from build123d import *

# Parameters (mm, degrees)
EXTRUDE_1_DEPTH          = 22
CUT_EXTRUDE_1_DEPTH      = 36.358874416
CUT_EXTRUDE_1_DEPTH_BACK = 36.358874416
SKETCH_3_W               = 15.710666492
SKETCH_3_H               = 11.25
SKETCH_3_W_2             = 17.010469835
SKETCH_3_H_2             = 12.25
SKETCH_4_R               = 2
CUT_EXTRUDE_2_DEPTH      = 52.983170353
PATTERN_LINEAR_1_COUNT   = 2
PATTERN_LINEAR_1_PITCH   = 23.5


with BuildPart() as part:
    # 草图1 → 凸台-拉伸1 (new, symmetric)
    with BuildSketch(Plane.XY):
        with BuildLine():
            Line((26.5, -8), (26.5, -6.486832981))
            ThreePointArc((26.5, -6.486832981), (26.461262373, -6.006286251), (26.346049894, -5.538149682))
            Line((26.346049894, -5.538149682), (25.183772234, -2.051316702))
            ThreePointArc((25.183772234, -2.051316702), (24.091853194, -0.566273444), (22.33772234, 0))
            Line((22.33772234, 0), (6.2, 0))
            ThreePointArc((6.2, 0), (-3.691899698, 4.980951377), (-1.803186005, -5.931991253))
            Line((-1.803186005, -5.931991253), (5, -8))
            Line((5, -8), (26.5, -8))
        make_face()
    extrude(amount=EXTRUDE_1_DEPTH, both=True)

    # 草图3 → 切除-拉伸1 (cut, two sides: drawn at the far end of the back side and taken through both)
    with BuildSketch(Plane(origin=(0, 0, 0), x_dir=(1, 0, 0), z_dir=(0, 1, 0)).offset(-CUT_EXTRUDE_1_DEPTH_BACK)):
        with Locations((-1.180894358, -16.375)):
            Rectangle(SKETCH_3_W, SKETCH_3_H)
        with Locations((-1.83079603, 5.625)):
            Rectangle(SKETCH_3_W_2, SKETCH_3_H_2)
    extrude(amount=CUT_EXTRUDE_1_DEPTH + CUT_EXTRUDE_1_DEPTH_BACK, mode=Mode.SUBTRACT)

    # 草图4 → 切除-拉伸2 (cut, through all)
    with BuildSketch(Plane(origin=(0, 0, -22), x_dir=(-1, 0, 0), z_dir=(0, 0, -1))):
        Circle(SKETCH_4_R)
    extrude(amount=-CUT_EXTRUDE_2_DEPTH, mode=Mode.SUBTRACT)

    # 草图5 → 切除-旋转1 (revolve, cut)
    with BuildSketch(Plane(origin=(0, 0, -11.75), x_dir=(-1, 0, 0), z_dir=(0, 0, -1))):
        Polygon((-15, 0), (-15, -8), (-11.75, -8), (-11.75, -6), (-9.2, -1), (-9.2, 0), align=None)
    cut_revolve_1 = revolve(axis=Axis((15, 0, -11.75), (0, -1, 0)), mode=Mode.SUBTRACT)

    # 阵列(线性)1: 切除-旋转1 ×2
    with Locations(*[(0, 0, i * PATTERN_LINEAR_1_PITCH) for i in range(1, PATTERN_LINEAR_1_COUNT)]):
        add(cut_revolve_1, mode=Mode.SUBTRACT)


solid = part.part
The model under review builds one solid part; all positions refer to its coordinate system, in mm. A direction names the side the tool comes from. Give positions to 0.01 mm unless a question says otherwise; leave off trailing zeros. Loops run counter-clockwise (first coordinate to the right, second up) from the corner with the lowest first, then second, coordinate; pieces in that order, holes last. Notation, with made-up numbers: (39.25, 83.5) -> (52.25, 83.5) arc R16 cw to (52.25, 87.5) -> close; hole circle Ø7 at (-8, 4). An arc over 180 degrees is marked (long way). Put each result on its own line as item: value. Start each with the question number.
1. For faces 4 (the face through (24.11, -0.58, 0.31)), 5 (the face through (0, -3, 10.75)), 6 (the face through (20.794, -0.493, 11.495)), list the 3-axis set-ups (+Z, -Z, +X, -X, +Y, -Y) from which the entire face can be reached by the end or side of a thin tool; tool diameter is ignored.
2. We need section D-D on y = 5.25. State the section outline as (x, z) points.
3. Wall thickness on probe 1 along Z at (x, y) = (15, -6.85); probe 2 along Z at (x, y) = (-4, 3); probe 3 along Z at (x, y) = (12.5, -1.5): over which ranges is each line inside the solid? List them lowest first.
4. Mouldability with a two-part tool opening along Z and no side actions: class faces 1 (the face through (14, 0, 0)), 2 (the face through (0, -3, 0.5)), 3 (the face through (10, -2, -22)) as released by +Z, released by -Z, zero draft, split by the parting line, or undercut.
5. We need section C-C on x = 0. State the section outline as (y, z) points, then the cut area to 3 significant figures.
6. Clearance check with flat-ended pins moving along their axes: P1, Ø10.5, axis at x = 15, z = -11.75, coming from the +Y side; P2, Ø6, axis at x = 12, z = -7, coming from the +Y side; P3, Ø2.5, axis at x = 0, y = 0, coming from the -Z side; P4, Ø4, axis at y = -5.5, z = -6.5, coming from the -X side. State where each tip first meets the part, or that it passes through.
7. We need section A-A on x = 15. State the section outline as (y, z) points.
8. We need section B-B on z = 11.75. State the section outline as (x, y) points, then the cut area to 3 significant figures.
Determined:
1. face 4: +Z, -Z, +X, +Y
1. face 5: +Z, -X, +Y, -Y
1. face 6: +Y
2. outline: (-3.3, -22) -> (3.3, -22) -> (3.3, -11.75) -> (-3.3, -11.75) -> close; (-3.3, 0.5) -> (3.3, 0.5) -> (3.3, 10.75) -> (-3.3, 10.75) -> close
3. probe 1: -22 to -15, -8.5 to 8.5, 15 to 22
3. probe 2: -22 to -11.75, 0.5 to 10.75
3. probe 3: -22 to -16.7, -6.8 to 6.8, 16.7 to 22
4. face 1: zero draft
4. face 2: undercut
4. face 3: released by -Z
5. outline: (-6.48, -22) -> (-2, -22) -> (-2, -11.75) -> (-6.48, -11.75) -> close; (-6.48, 0.5) -> (-2, 0.5) -> (-2, 10.75) -> (-6.48, 10.75) -> close; (2, -22) -> (6.2, -22) -> (6.2, -11.75) -> (2, -11.75) -> close; (2, 0.5) -> (6.2, 0.5) -> (6.2, 10.75) -> (2, 10.75) -> close
5. area: 178 mm^2
6. P1: y = -2.08
6. P2: y = 0
6. P3: through
6. P4: x = 6.67
7. outline: (-8, -22) -> (0, -22) -> (0, -17.55) -> (-1, -17.55) -> (-6, -15) -> (-8, -15) -> close; (-8, -8.5) -> (-6, -8.5) -> (-1, -5.95) -> (0, -5.95) -> (0, 5.95) -> (-1, 5.95) -> (-6, 8.5) -> (-8, 8.5) -> close; (-8, 15) -> (-6, 15) -> (-1, 17.55) -> (0, 17.55) -> (0, 22) -> (-8, 22) -> close
8. outline: (6.67, -8) -> (11.75, -8) -> (11.75, -6) -> (9.2, -1) -> (9.2, 0) -> (6.67, 0) -> close; (18.25, -8) -> (26.5, -8) -> (26.5, -6.49) arc R3 ccw to (26.35, -5.54) -> (25.18, -2.05) arc R3 ccw to (22.34, 0) -> (20.8, 0) -> (20.8, -1) -> (18.25, -6) -> close
8. area: 81.9 mm^2
